Read the model definition and answer for the solid it produces. Units are mm, in the model's axes. Give positions to 0.01 mm unless a question says otherwise; leave off trailing zeros. Order: outer loops, then holes, each group sorted by start corner. A loop starts at its lowest first (then second) coordinate and runs counter-clockwise, first axis right, second up.
Item 1: Given pin 1 Ø4 at (x, y) = (3.75, -30) entering from -Z; pin 2 Ø1.9 at (x, y) = (-3.75, 30) entering from -Z, each flat-ended and moving along its own axis, determine where each tip first touches the part or whether it passes through.
Item 2: Find the intervals of material crossed by line 1 along Y through (x, z) = (-3.75, 4.85); line 2 along Z through (x, y) = (2, -38); line 3 along X through (y, z) = (-65.5, 4.2), in increasing order.
Item 3: A cutting plane is placed at C-C (z = -2). Write down the section's boundary in (x, y).
Item 4: A cutting plane is placed at B-B (y = 45.5). Write down the section's boundary in (x, z), plus the area to 3 significant figures.
Item 5: A cutting plane is placed at D-D (y = 26). Write down the section's boundary in (x, z), plus the area to 3 significant figures.
Item 6: A cutting plane is placed at A-A (x = -3.75). Write down the section's boundary in (y, z), plus the area to 3 significant figures.
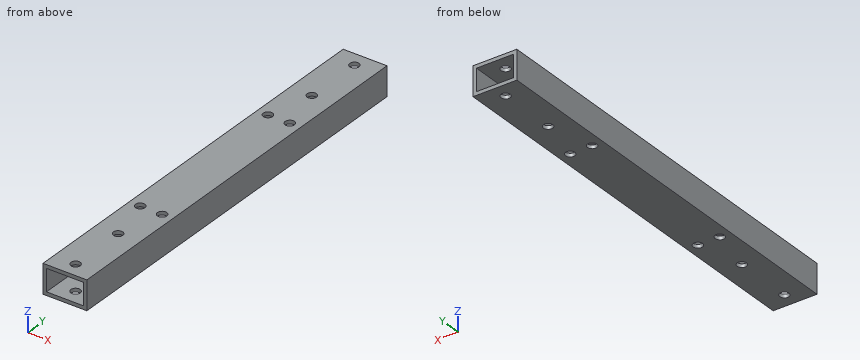
from build123d import *

# Parameters (mm, degrees)
SKETCH_1_W          = 15
SKETCH_1_H          = 10
SKETCH_1_W_2        = 12.6
SKETCH_1_H_2        = 7.6
EXTRUDE_1_DEPTH     = 70.5
SKETCH_2_R          = 1.6
CUT_EXTRUDE_1_DEPTH = 100


with BuildPart() as part:
    # ｽｹｯﾁ1 → ﾎﾞｽ - 押し出し1 (new, symmetric)
    with BuildSketch(Plane(origin=(0, 0, 0), x_dir=(1, 0, 0), z_dir=(0, 1, 0))):
        Rectangle(SKETCH_1_W, SKETCH_1_H)
        Rectangle(SKETCH_1_W_2, SKETCH_1_H_2, mode=Mode.SUBTRACT)
    extrude(amount=EXTRUDE_1_DEPTH, both=True)

    # ｽｹｯﾁ2 → ｶｯﾄ - 押し出し1 (cut)
    with BuildSketch(Plane(origin=(0, 0, -5), x_dir=(-1, 0, 0), z_dir=(0, 0, -1))):
        with Locations((0, -65.5)):
            Circle(SKETCH_2_R)
        with Locations((0, -45.5)):
            Circle(SKETCH_2_R)
        with Locations(Location((0, 45.5, 0), (0, 0, 180))):
            Circle(SKETCH_2_R)
        with Locations(Location((0, 65.5, 0), (0, 0, 180))):
            Circle(SKETCH_2_R)
        with Locations((3.75, -30)):
            Circle(SKETCH_2_R)
        with Locations(Location((-3.75, -30, 0), (0, 0, 180))):
            Circle(SKETCH_2_R)
        with Locations((-3.75, 30)):
            Circle(SKETCH_2_R)
        with Locations(Location((3.75, 30, 0), (0, 0, 180))):
            Circle(SKETCH_2_R)
    extrude(amount=-CUT_EXTRUDE_1_DEPTH, mode=Mode.SUBTRACT)


solid = part.part
Response values:
1. pin 1: stops at z = -5
1. pin 2: passes through
2. line 1: y = -70.5 to -31.6, -28.4 to 28.4, 31.6 to 70.5
2. line 2: z = -5 to -3.8, 3.8 to 5
2. line 3: x = -7.5 to -1.6, 1.6 to 7.5
3. outline: (-7.5, -70.5) - (-6.3, -70.5) - (-6.3, 70.5) - (-7.5, 70.5) - close; (6.3, -70.5) - (7.5, -70.5) - (7.5, 70.5) - (6.3, 70.5) - close
4. outline: (-7.5, -5) - (-1.6, -5) - (-1.6, -3.8) - (-6.3, -3.8) - (-6.3, 3.8) - (-1.6, 3.8) - (-1.6, 5) - (-7.5, 5) - close; (1.6, -5) - (7.5, -5) - (7.5, 5) - (1.6, 5) - (1.6, 3.8) - (6.3, 3.8) - (6.3, -3.8) - (1.6, -3.8) - close
4. area: 46.6 mm2
5. outline: (-7.5, -5) - (7.5, -5) - (7.5, 5) - (-7.5, 5) - close; hole (-6.3, -3.8) - (6.3, -3.8) - (6.3, 3.8) - (-6.3, 3.8) - close
5. area: 54.2 mm2
6. outline: (-70.5, -5) - (-31.6, -5) - (-31.6, -3.8) - (-70.5, -3.8) - close; (-70.5, 3.8) - (-31.6, 3.8) - (-31.6, 5) - (-70.5, 5) - close; (-28.4, -5) - (28.4, -5) - (28.4, -3.8) - (-28.4, -3.8) - close; (-28.4, 3.8) - (28.4, 3.8) - (28.4, 5) - (-28.4, 5) - close; (31.6, -5) - (70.5, -5) - (70.5, -3.8) - (31.6, -3.8) - close; (31.6, 3.8) - (70.5, 3.8) - (70.5, 5) - (31.6, 5) - close
6. area: 323 mm2
